from build123d import *

# Parameters (mm, degrees)
BOSS_EXTRUDE1_DEPTH = 3.175
FILLET1_R           = 3.175
FILLET2_R           = 15.875
SKETCH2_R           = 1.5875
CUT_EXTRUDE1_DEPTH  = 228.228874156
SKETCH3_R           = 2.5273
CUT_EXTRUDE2_DEPTH  = 228.228874156
SKETCH4_R           = 2.5273
CUT_EXTRUDE3_DEPTH  = 228.228874156
SKETCH7_R           = 1.524
CUT_EXTRUDE6_DEPTH  = 228.228874156
SKETCH8_R           = 1.524
CUT_EXTRUDE7_DEPTH  = 228.228874156
SKETCH10_W          = 25.4
SKETCH10_H          = 3.048
CUT_EXTRUDE9_DEPTH  = 228.228874156
SKETCH11_W          = 49.53
SKETCH11_H          = 3.81
CUT_EXTRUDE10_DEPTH = 228.228874156


with BuildPart() as part:
    # Sketch1 → Boss-Extrude1 (new body)
    with BuildSketch(Plane(origin=(0, 0, 0), x_dir=(1, 0, 0), z_dir=(0, 1, 0))):
        Polygon((0, 102.87), (0, 158.75), (38.1, 158.75), (38.1, 190.5), (69.85, 190.5), (69.85, 158.75), (107.95, 158.75), (107.95, 102.87), (123.825, 102.87), (123.825, 55.88), (107.95, 55.88), (107.95, 0), (69.85, 0), (69.85, -31.75), (38.1, -31.75), (38.1, 0), (0, 0), (0, 55.88), (-15.875, 55.88), (-15.875, 102.87), align=None)
    extrude(amount=BOSS_EXTRUDE1_DEPTH)

    # Fillet1
    fillet1_edges = [part.edges().sort_by_distance(p)[0] for p in [
        (0, 1.5875, -55.88),
        (0, 1.5875, -102.87),
        (0, 1.5875, -158.75),
        (38.1, 1.5875, -158.75),
        (69.85, 1.5875, -158.75),
        (107.95, 1.5875, -158.75),
        (107.95, 1.5875, -102.87),
        (107.95, 1.5875, -55.88),
        (107.95, 1.5875, 0),
        (69.85, 1.5875, 0),
        (38.1, 1.5875, 0),
        (0, 1.5875, 0),
    ]]
    fillet(fillet1_edges, radius=FILLET1_R)

    # Fillet2
    fillet2_edges = [part.edges().sort_by_distance(p)[0] for p in [
        (38.1, 1.5875, 31.75),
        (69.85, 1.5875, 31.75),
        (69.85, 1.5875, -190.5),
        (38.1, 1.5875, -190.5),
    ]]
    fillet(fillet2_edges, radius=FILLET2_R - 0.0001)  # a hair under: the kernel refuses the full size

    # Sketch2 → Cut-Extrude1 (cut, through all)
    with BuildSketch(Plane(origin=(0, 3.175, 0), x_dir=(1, 0, 0), z_dir=(0, 1, 0))):
        with Locations(Location((53.975, 180.34, 0), (0, 0, 270))):
            Circle(SKETCH2_R)
        with Locations(Location((53.975, -21.59, 0), (0, 0, 270))):
            Circle(SKETCH2_R)
    extrude(amount=-CUT_EXTRUDE1_DEPTH, mode=Mode.SUBTRACT)

    # Sketch3 → Cut-Extrude2 (cut, through all)
    with BuildSketch(Plane.XZ):
        with Locations(Location((-6.35, -68.326, 0), (0, 0, 270))):
            Circle(SKETCH3_R)
        with Locations(Location((-6.35, -90.424, 0), (0, 0, 270))):
            Circle(SKETCH3_R)
        with Locations(Location((114.3, -68.326, 0), (0, 0, 270))):
            Circle(SKETCH3_R)
        with Locations(Location((114.3, -90.424, 0), (0, 0, 270))):
            Circle(SKETCH3_R)
    extrude(amount=-CUT_EXTRUDE2_DEPTH, mode=Mode.SUBTRACT)

    # Sketch4 → Cut-Extrude3 (cut, through all)
    with BuildSketch(Plane.XZ):
        with Locations(Location((52.959, -56.261, 0), (0, 0, 270))):
            Circle(SKETCH4_R)
        with Locations(Location((52.959, -104.013, 0), (0, 0, 270))):
            Circle(SKETCH4_R)
    extrude(amount=-CUT_EXTRUDE3_DEPTH, mode=Mode.SUBTRACT)

    # Sketch7 → Cut-Extrude6 (cut, through all)
    with BuildSketch(Plane.XZ):
        with Locations(Location((32.87141, -49.784, 0), (0, 0, 270))):
            Circle(SKETCH7_R)
    extrude(amount=-CUT_EXTRUDE6_DEPTH, mode=Mode.SUBTRACT)

    # Sketch8 → Cut-Extrude7 (cut, through all)
    with BuildSketch(Plane.XZ):
        with Locations(Location((35.60064, -116.9416, 0), (0, 0, 270))):
            Circle(SKETCH8_R)
        with Locations(Location((35.60064, -155.0416, 0), (0, 0, 270))):
            Circle(SKETCH8_R)
        with Locations(Location((72.9996, -116.9416, 0), (0, 0, 270))):
            Circle(SKETCH8_R)
        with Locations(Location((72.9996, -155.0416, 0), (0, 0, 270))):
            Circle(SKETCH8_R)
    extrude(amount=-CUT_EXTRUDE7_DEPTH, mode=Mode.SUBTRACT)

    # Sketch10 → Cut-Extrude9 (cut, through all)
    with BuildSketch(Plane.XZ):
        with Locations((25.4, -38.1)):
            Rectangle(SKETCH10_W, SKETCH10_H)
    extrude(amount=-CUT_EXTRUDE9_DEPTH, mode=Mode.SUBTRACT)

    # Sketch11 → Cut-Extrude10 (cut, through all)
    with BuildSketch(Plane.XZ):
        with Locations((27.305, -5.715)):
            Rectangle(SKETCH11_W, SKETCH11_H)
        with Locations((27.305, -30.353)):
            Rectangle(SKETCH11_W, SKETCH11_H)
        with Locations((80.645, -5.715)):
            Rectangle(SKETCH11_W, SKETCH11_H)
        with Locations((80.645, -30.353)):
            Rectangle(SKETCH11_W, SKETCH11_H)
    extrude(amount=-CUT_EXTRUDE10_DEPTH, mode=Mode.SUBTRACT)


solid = part.part
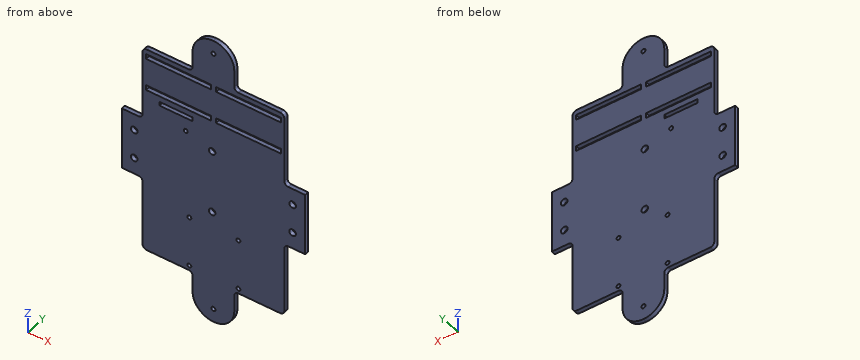
Build history of the part. All positions in model axes, mm. Coordinates: 2 decimals unless noted, no trailing zeros. Order: outer loops, then holes, each group sorted by start corner. A loop starts at its lowest first (then second) coordinate and runs counter-clockwise, first axis right, second up. Notation, with made-up numbers: M 46,85.5 L 83,85.5 A25 ccw 83,111.5 Z; hole C -32,-35.75 d9. An arc over 180 degrees is marked long. One line per question, with ' | ' between items. Start each with the question number.
Q1. Saw through at A-A (x = 114.3). List the corners of the cut face in (y, z) (3 decimals).
Q2. Saw through at C-C (z = -141). List the corners of the cut face in (x, y) (3 decimals), then the cut area to 3 significant figures.
Q3. Probe L1, parallel to Z at x = 14, y = 1.45; L2, parallel to Z at x = 81, y = 0.35; L3, parallel to Z at x = 73, y = 0.55. List the from-to ranges inside material, lowest first. Write a range as from..to.
Q4. Flat gauge pins, fed straight in: pin 1 Ø1.6 at (x, y) = (116.5, 1.5) entering from +Z; pin 2 Ø1 at (y, z) = (1, -29.5) entering from +X; pin 3 Ø1 at (x, y) = (12.5, 2) entering from -Z. Where does each tip first touch, or does it go through?
Q5. Saw through at D-D (y = 1.95). Count the separate pieces of the cut face and the enclosed holes in it, then the cut area to 3 significant figures.
Q6. Saw through at B-B (x = 84). List the corners of the cut face in (y, z) (3 decimals), then the cut area to 3 significant figures.
Check values:
1) outline: M 0,-102.87 L 3.175,-102.87 L 3.175,-92.951 L 0,-92.951 Z; M 0,-87.897 L 3.175,-87.897 L 3.175,-70.853 L 0,-70.853 Z; M 0,-65.799 L 3.175,-65.799 L 3.175,-55.88 L 0,-55.88 Z
2) outline: M 0,0 L 107.95,0 L 107.95,3.175 L 0,3.175 Z | area: 343 mm2
3) L1: z = -158.75..-39.62, -36.58..-32.26, -28.45..-7.62, -3.81..0 | L2: z = -158.75..-32.26, -28.45..-7.62, -3.81..0 | L3: z = -158.75..-156.57, -153.52..-118.47, -115.42..-32.26, -28.45..-7.62, -3.81..0
4) pin 1: stops at z = -55.88 | pin 2: stops at x = 107.95 | pin 3: stops at z = -158.75
5) separate pieces: 1 | enclosed holes: 18 | area: 19,400 mm2
6) outline: M 0,-158.75 L 3.175,-158.75 L 3.175,-32.258 L 0,-32.258 Z; M 0,-28.448 L 3.175,-28.448 L 3.175,-7.62 L 0,-7.62 Z; M 0,-3.81 L 3.175,-3.81 L 3.175,0 L 0,0 Z | area: 480 mm2
